Geometry: final body of the model. Coordinates: model frame, mm. A direction names the side the tool comes from. Coordinates: 2 decimals unless noted, no trailing zeros. Loops run counter-clockwise (first coordinate to the right, second up) from the corner with the lowest first, then second, coordinate; pieces in that order, holes last. Notation, with made-up numbers: (-5, 28) - (27, 28) arc R30 cw to (27, 56) - close; hole circle Ø8 at (67, -11.5). An arc over 180 degrees is marked (long way). Answer in a Markdown table with one row per item.
from build123d import *

# Parameters (mm, degrees)
F0_W     = 60
F0_H     = 40
F1_DEPTH = 35
F2_W     = 54
F2_H     = 34
F3_DEPTH = 32
F5_DEPTH = 5
F7_DEPTH = 5


with BuildPart() as f1:
    # F0 (on Top) → F1 (new body)
    with BuildSketch(Plane.XY):
        with Locations((-0.1621283591, -0.2469897495)):
            Rectangle(F0_W, F0_H)
    extrude(amount=F1_DEPTH)

    # F2 (on face) → F3 (cut)
    with BuildSketch(Plane.XY.offset(35)):
        with Locations((-0.1621283591, -0.2469897495)):
            Rectangle(F2_W, F2_H)
    extrude(amount=-F3_DEPTH, mode=Mode.SUBTRACT)

    # F4 (on face) → F5 (cut)
    with BuildSketch(Plane(origin=(-30.1621283591, 0, 0), x_dir=(0, -1, 0), z_dir=(-1, 0, 0))):
        with BuildLine():
            Line((0, 35), (-6.551516708, 35))
            add(Edge.make_bspline(
                [(-6.551516708, 35), (-5.8386453378, 30.8886812927), (-4.389754715, 22.5325438864), (-1.4787538932, 30.8001527505), (0, 35)],
                knots=[0, 0, 0, 0, 0.49201186, 1, 1, 1, 1], degree=3))
        make_face()
    extrude(amount=-F5_DEPTH, mode=Mode.SUBTRACT)

    # F6 (on face) → F7 (cut)
    with BuildSketch(Plane.YZ.offset(29.8378716409)):
        with BuildLine():
            Line((13.9640960842, 35), (7.9849697649, 35))
            add(Edge.make_bspline(
                [(7.9849697649, 35), (9.0646587158, 31.5158458238), (11.2144741419, 24.578395562), (13.0502773485, 31.5364484313), (13.9640960842, 35)],
                knots=[0, 0, 0, 0, 0.5022240225, 1, 1, 1, 1], degree=3))
        make_face()
    extrude(amount=-F7_DEPTH, mode=Mode.SUBTRACT)


solid = f1.part
(1) Pull-direction query (X, two-part tool) for faces 3 (the face through (-30.162, -1, 17)), 4 (the face through (29.838, -1, 17)), 5 (the face through (26.838, 0, 19)), 6 (the face through (2, -18, 35)); classes: pulls with the +X half, pulls with the -X half, needs draft (parallel to the pull), parting line crosses it, or undercut.
Verdict:
| item | result |
|---|---|
| face 3 | pulls with the -X half |
| face 4 | pulls with the +X half |
| face 5 | undercut |
| face 6 | needs draft |
(2) First-contact query: pin 1 Ø2 at (x, y) = (-21, 12.5) entering from -Z; pin 2 Ø12 at (x, y) = (0.5, -7) entering from +Z. Flat tips, straight axial feed; report the tip coordinate or a pass-through.
Verdict:
| item | result |
|---|---|
| pin 1 | stops at z = 0 |
| pin 2 | stops at z = 3 |
(3) Ray query, probe 1 along Y at (x, z) = (22, 19); probe 2 along X at (y, z) = (-0.5, 13); probe 3 along Z at (x, y) = (-12, -17). Return the intervals inside material, ascending.
Verdict:
| item | result |
|---|---|
| probe 1 | y = -20.25 to -17.25, 16.75 to 19.75 |
| probe 2 | x = -30.16 to -27.16, 26.84 to 29.84 |
| probe 3 | z = 0 to 3 |
(4) Cut plane B-B on z = 22. Output: boundary loops of the cut face in (x, y).
Verdict:
| item | result |
|---|---|
| outline | (-30.16, -20.25) - (29.84, -20.25) - (29.84, 19.75) - (-30.16, 19.75) - close; hole (-27.16, -17.25) - (26.84, -17.25) - (26.84, 16.75) - (-27.16, 16.75) - close |
(5) Cut plane A-A on x = -15. Output: boundary loops of the cut face in (y, z), then the cut area to 3 significant figures.
Verdict:
| item | result |
|---|---|
| outline | (-20.25, 0) - (19.75, 0) - (19.75, 35) - (16.75, 35) - (16.75, 3) - (-17.25, 3) - (-17.25, 35) - (-20.25, 35) - close |
| area | 312 mm² |
(6) Cut plane C-C on y = -6.5. Output: boundary loops of the cut face in (x, z), then the cut area to 3 significant figures.
Verdict:
| item | result |
|---|---|
| outline | (-30.16, 0) - (29.84, 0) - (29.84, 35) - (26.84, 35) - (26.84, 3) - (-27.16, 3) - (-27.16, 35) - (-30.16, 35) - close |
| area | 372 mm² |
(7) Access query for faces 1 (the face through (-3, 18, 35)), 2 (the face through (-27.162, 0, 19)). Directions: +Z, -Z, +X, -X, +Y, -Y. A direction counts if a zero-diameter tool reaches every point of the face in a straight line with its end or side. Return the directions, or none.
Verdict:
| item | result |
|---|---|
| face 1 | +Z, +X, -X, +Y, -Y |
| face 2 | +Z |
